Check sheet for the modelled part. Datum: model origin and axes. Units: mm. Coordinates: 2 decimals unless noted, no trailing zeros. Loops run counter-clockwise (first coordinate to the right, second up) from the corner with the lowest first, then second, coordinate; pieces in that order, holes last. Notation, with made-up numbers: M -26,-39 L 5,-39 A23 ccw 5,-27 Z; hole C 40.5,30.25 d9. An arc over 180 degrees is marked long. Answer in a Markdown table with one row per item. Add a question column.
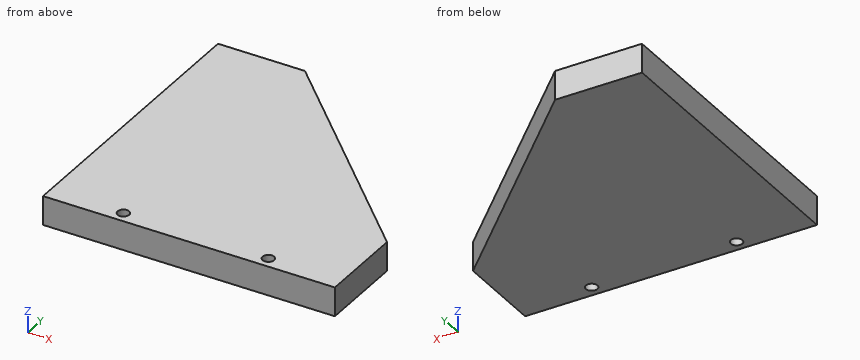
```python
from build123d import *

# Parameters (mm, degrees)
BOSS_EXTRU_1_DEPTH           = 10
ENL_V_MAT_EXTRU_1_DEPTH      = 143.777033777
ENL_V_MAT_EXTRU_1_DEPTH_BACK = 143.777033777
ESQUISSE2_R                  = 2


with BuildPart() as part:
    # Esquisse1 → Boss.-Extru.1 (new body)
    with BuildSketch(Plane.XY):
        Polygon((0, 0), (0, 100.710678119), (30, 100.710678119), (100.710678119, 30), (100.710678119, 0), align=None)
    extrude(amount=BOSS_EXTRU_1_DEPTH)

    # Esquisse2 → Enlèv. mat.-Extru.1 (cut, two sides: drawn at the far end of the back side and taken through both)
    with BuildSketch(Plane.XY.offset(10).offset(-ENL_V_MAT_EXTRU_1_DEPTH_BACK)):
        with Locations((25.355339059, 4)):
            Circle(ESQUISSE2_R)
        with Locations(Location((75.355339059, 4, 0), (0, 0, 180))):
            Circle(ESQUISSE2_R)
    extrude(amount=ENL_V_MAT_EXTRU_1_DEPTH + ENL_V_MAT_EXTRU_1_DEPTH_BACK, mode=Mode.SUBTRACT)


solid = part.part
```
Q1. Cross-section at B-B (z = 6). Record the cut outline in (x, y).
Q2. Cross-section at D-D (y = 42). Record the cut outline in (x, z), plus the area to 3 significant figures.
Q3. Cross-section at A-A (y = 4). Record the cut outline in (x, z), plus the area to 3 significant figures.
Q4. Cross-section at C-C (x = 26). Record the cut outline in (y, z), plus the area to 3 significant figures.
Q5. Thickness scan on L1, parallel to Y at x = 74.5, z = 5.5; L2, parallel to Y at x = 53.5, z = 7; L3, parallel to Y at x = 44.5, z = 7.75. Record the ranges inside material, lowest first.
Q6. Go/stop test with a flat-tipped pin: pin 1 (5 mm diameter, centred on x = 73.5, z = 2.5, fed in from +Y). Record where the tip stops, or that it passes through.
Answer key:
| question | item | result |
|---|---|---|
| 1 | outline | M 0,0 L 100.71,0 L 100.71,30 L 30,100.71 L 0,100.71 Z; hole C 25.36,4 d4; hole C 75.36,4 d4 |
| 2 | outline | M 0,0 L 88.71,0 L 88.71,10 L 0,10 Z |
| 2 | area | 887 mm^2 |
| 3 | outline | M 0,0 L 23.36,0 L 23.36,10 L 0,10 Z; M 27.36,0 L 73.36,0 L 73.36,10 L 27.36,10 Z; M 77.36,0 L 100.71,0 L 100.71,10 L 77.36,10 Z |
| 3 | area | 927 mm^2 |
| 4 | outline | M 0,0 L 2.11,0 L 2.11,10 L 0,10 Z; M 5.89,0 L 100.71,0 L 100.71,10 L 5.89,10 Z |
| 4 | area | 969 mm^2 |
| 5 | L1 | 0 to 2.19, 5.81 to 56.21 |
| 5 | L2 | 0 to 77.21 |
| 5 | L3 | 0 to 86.21 |
| 6 | pin 1 | y = 59.71 |
